Verification items for the finished model (mm, model axes). Face numbers are marked on the shaded views. Round coordinates to 2 decimals unless told otherwise and drop trailing zeros. Order: outer loops, then holes, each group sorted by start corner. A loop starts at its lowest first (then second) coordinate and runs counter-clockwise, first axis right, second up. Notation, with made-up numbers: M 43,72 L 66,72 A21 ccw 66,81 Z; hole C 36.5,85 d1. An arc over 180 degrees is marked long. Answer as a JSON object with one key per item and string values. Group by question number.
```python
from build123d import *

# Parameters (mm, degrees)
ESQUISSE1_R             = 51.1
BOSS_EXTRU_1_DEPTH      = 11.482
CUT_EXTRUDE1_DEPTH      = 107.685689406
CUT_EXTRUDE1_DEPTH_BACK = 107.685689406
SKETCH1_R               = 1.6


with BuildPart() as part:
    # Esquisse1 → Boss.-Extru.1 (new body)
    with BuildSketch(Plane(origin=(0, 0, 0), x_dir=(0, 0, -1), z_dir=(1, 0, 0))):
        with BuildLine():
            Line((-5.741, 64.1), (-5.741, 74.77994998))
            ThreePointArc((-5.741, 74.77994998), (-64.951905284, 37.5), (-67.631836376, -32.418123147))
            Line((-67.631836376, -32.418123147), (-58.382728383, -27.078148157))
            Line((-58.382728383, -27.078148157), (-52.641728383, -37.021851843))
            Line((-52.641728383, -37.021851843), (-61.890836376, -42.361826833))
            ThreePointArc((-61.890836376, -42.361826833), (0, -75), (61.890836376, -42.361826833))
            Line((61.890836376, -42.361826833), (52.641728383, -37.021851843))
            Line((52.641728383, -37.021851843), (58.382728383, -27.078148157))
            Line((58.382728383, -27.078148157), (67.631836376, -32.418123147))
            ThreePointArc((67.631836376, -32.418123147), (64.951905284, 37.5), (5.741, 74.77994998))
            Line((5.741, 74.77994998), (5.741, 64.1))
            Line((5.741, 64.1), (-5.741, 64.1))
        make_face()
        Circle(ESQUISSE1_R, mode=Mode.SUBTRACT)
    extrude(amount=BOSS_EXTRU_1_DEPTH)

    # Sketch1 → Cut-Extrude1 (cut, two sides: drawn at the far end of the back side and taken through both)
    with BuildSketch(Plane(origin=(0, 0, 0), x_dir=(0, 0, -1), z_dir=(1, 0, 0)).offset(-CUT_EXTRUDE1_DEPTH_BACK)):
        with Locations((22.573329459, 62.019712972)):
            Circle(SKETCH1_R)
        with Locations((57.15767665, 33)):
            Circle(SKETCH1_R)
        with Locations((64.997311699, -11.460779726)):
            Circle(SKETCH1_R)
        with Locations((42.423982239, -50.558933246)):
            Circle(SKETCH1_R)
        with Locations((0, -66)):
            Circle(SKETCH1_R)
        with Locations((-42.423982239, -50.558933246)):
            Circle(SKETCH1_R)
        with Locations((-64.997311699, -11.460779726)):
            Circle(SKETCH1_R)
        with Locations((-57.15767665, 33)):
            Circle(SKETCH1_R)
        with Locations((-22.573329459, 62.019712972)):
            Circle(SKETCH1_R)
    extrude(amount=CUT_EXTRUDE1_DEPTH + CUT_EXTRUDE1_DEPTH_BACK, mode=Mode.SUBTRACT)


solid = part.part
```
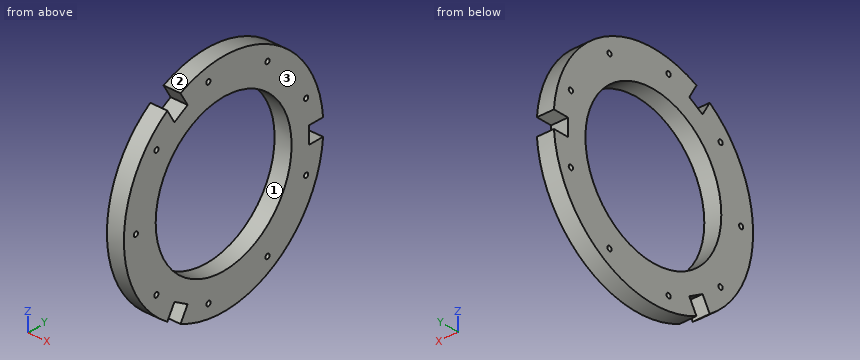
Q1. Release check for a two-part mould opening along Z. For the marked faces 1, 2 and 3 record: released by +Z, released by -Z, zero draft, split by the parting line, or undercut.
Q2. Gauge pin test, flat ends, axial feed: pin 1 Ø6 at (x, z) = (4.5, 58.5) entering from +Y; pin 2 Ø5 at (x, z) = (9, -36) entering from -Y; pin 3 Ø6 at (x, z) = (10, -28.5) entering from -Y. Record the tip position at first contact, or that the pin passes through.
Q3. Thickness scan on line 1 (Y direction, x = 1.5, z = -24); line 2 (Z direction, x = 0.5, y = 62.5); line 3 (Z direction, x = 5.5, y = 62). Record the ranges inside material, lowest first. Write a range as from..to.
Q4. Cross-section at A-A, the plane y = 0. Record the cut outline in (x, z).
Q5. Cross-section at B-B, the plane z = 18. Record the cut outline in (x, y).
Q6. Cross-section at C-C, the plane x = 4.25. Give the number of separate pieces and of enclosed holes in the cut face, then the cut area to 3 significant figures.
Conclusion:
{
 "1": {"face 1": "undercut", "face 2": "released by +Z", "face 3": "zero draft"},
 "2": {"pin 1": "y = 50.45", "pin 2": "y = -67.1", "pin 3": "y = -70.53"},
 "3": {"line 1": "-71.06..-45.11, 45.11..61.3, 62.74..71.06", "line 2": "-41.46..-24.1, -21.05..21.05, 24.1..41.46", "line 3": "-42.2..-24.17, -20.97..20.97, 24.17..42.2"},
 "4": {"outline": "M 0,-75 L 11.48,-75 L 11.48,-51.1 L 0,-51.1 Z; M 0,51.1 L 11.48,51.1 L 11.48,75 L 0,75 Z"},
 "5": {"outline": "M 0,-72.81 L 11.48,-72.81 L 11.48,-47.82 L 0,-47.82 Z; M 0,47.82 L 11.48,47.82 L 11.48,72.81 L 0,72.81 Z"},
 "6": {"separate pieces": "1", "enclosed holes": "10", "area": "9,020 mm2"}
}
